from build123d import *

# Parameters (mm, degrees)
SKETCH1_R                                = 4.25
BOSS_EXTRUDE1_DEPTH                      = 10
BOSS_EXTRUDE2_START                      = -5
BOSS_EXTRUDE2_DEPTH                      = 15
SKETCH3_W                                = 342
SKETCH3_H                                = 10
BOSS_EXTRUDE3_DEPTH                      = 304
CUT_EXTRUDE1_REACH                       = 385.234
BOSS_EXTRUDE4_DEPTH                      = 3
MIRROR5_AT_THE_SECOND_PLANE_COPY_1_DEPTH = 3
BOSS_EXTRUDE5_DEPTH                      = 5
BOSS_EXTRUDE5_DEPTH_BACK                 = 5
BOSS_EXTRUDE6_DEPTH                      = 10
SKETCH10_W                               = 19
SKETCH10_H                               = 21.5
SKETCH10_R                               = 4.25
BOSS_EXTRUDE7_DEPTH                      = 10
CUT_EXTRUDE2_REACH                       = 276.29
SKETCH11_W                               = 2.5
SKETCH11_H                               = 70
MIRROR8_COPY_1_DEPTH                     = 10
MIRROR8_COPY_2_DEPTH                     = 10
MIRROR8_COPY_3_SKETCH_W                  = 19
MIRROR8_COPY_3_SKETCH_H                  = 21.5
MIRROR8_COPY_3_SKETCH_R                  = 4.25
MIRROR8_COPY_3_DEPTH                     = 10
CUT_EXTRUDE5_REACH                       = 415.459
SKETCH14_W                               = 574.948758302
SKETCH14_H                               = 178.61459587
CUT_EXTRUDE6_REACH                       = 276.29
SKETCH15_W                               = 297.993149394
SKETCH15_H                               = 172.333387601


with BuildPart() as part:
    # Sketch1 → Boss-Extrude1 (new body)
    with BuildSketch(Plane(origin=(0, 0, 0), x_dir=(1, 0, 0), z_dir=(0, 1, 0))):
        Polygon((-171, 12.5), (171, 12.5), (171, 0), (171, -12.5), (158, -12.5), (158, 0), (-158, 0), (-158, -12.5), (-171, -12.5), align=None)
        with Locations(Location((-145.5, 6.25, 0), (0, 0, 270))):
            Circle(SKETCH1_R, mode=Mode.SUBTRACT)
        with Locations(Location((145.5, 6.25, 0), (0, 0, 90))):
            Circle(SKETCH1_R, mode=Mode.SUBTRACT)
        with Locations(Location((-25.5, 6.25, 0), (0, 0, 270))):
            Circle(SKETCH1_R, mode=Mode.SUBTRACT)
        with Locations(Location((25.5, 6.25, 0), (0, 0, 270))):
            Circle(SKETCH1_R, mode=Mode.SUBTRACT)
    boss_extrude1 = extrude(amount=BOSS_EXTRUDE1_DEPTH)

    # Sketch2 → Boss-Extrude2 (add)
    with BuildSketch(Plane.XY.offset(12.5).offset(BOSS_EXTRUDE2_START)):
        Polygon((-171, 105), (-171, 0), (-158, 0), (-158, 80), (158, 80), (158, 0), (171, 0), (171, 105), align=None)
    boss_extrude2 = extrude(amount=BOSS_EXTRUDE2_DEPTH)

    # Sketch3 → Boss-Extrude3 (add)
    with BuildSketch(Plane.XY.offset(22.5)):
        with Locations((0, 85)):
            Rectangle(SKETCH3_W, SKETCH3_H)
    extrude(amount=BOSS_EXTRUDE3_DEPTH)

    # Sketch4 → Cut-Extrude1 (cut, up to next)
    with BuildSketch(Plane(origin=(0, 105, 0), x_dir=(1, 0, 0), z_dir=(0, 1, 0)), mode=Mode.PRIVATE) as cut_extrude1_sk1:
        Polygon((-163.5, -22.5), (-5, -22.5), (-5, -326.5), (-163.5, -326.5), (-163.5, -39.75), (-163.5, -34.75), align=None)
    cut_extrude1_tool1 = extrude(cut_extrude1_sk1.sketch, amount=-CUT_EXTRUDE1_REACH, mode=Mode.PRIVATE) & part.part
    # Sketch4 → Cut-Extrude1 (cut, up to next)
    with BuildSketch(Plane(origin=(0, 105, 0), x_dir=(1, 0, 0), z_dir=(0, 1, 0)), mode=Mode.PRIVATE) as cut_extrude1_sk2:
        Polygon((163.5, -22.5), (163.5, -51.4723011), (163.5, -326.5), (5, -326.5), (5, -39.75), (5, -22.5), align=None)
    cut_extrude1_tool2 = extrude(cut_extrude1_sk2.sketch, amount=-CUT_EXTRUDE1_REACH, mode=Mode.PRIVATE) & part.part
    add(cut_extrude1_tool1.solids().sort_by_distance((-84.25, 105, 174.5))[0], mode=Mode.SUBTRACT)
    add(cut_extrude1_tool2.solids().sort_by_distance((84.25, 105, 174.5))[0], mode=Mode.SUBTRACT)

    # Mirror3: Boss-Extrude2 across plane
    add(boss_extrude2.mirror(Plane(origin=(0, 0, 174.5), x_dir=(1, 0, 0), z_dir=(0, 0, -1))))

    # Mirror4: Boss-Extrude1 across plane
    add(boss_extrude1.mirror(Plane(origin=(0, 0, 174.5), x_dir=(1, 0, 0), z_dir=(0, 0, -1))))

    # Sketch7 → Boss-Extrude4 (add)
    with BuildSketch(Plane(origin=(0, 80, 0), x_dir=(-1, 0, 0), z_dir=(0, -1, 0))):
        Polygon((-163.5, -22.5), (-148.5, -22.5), (-163.5, -37.5), align=None)
        Polygon((-5, -22.5), (-20, -22.5), (-5, -37.5), align=None)
    boss_extrude4 = extrude(amount=-BOSS_EXTRUDE4_DEPTH)

    # Mirror5: Boss-Extrude4 across plane
    add(boss_extrude4.mirror(Plane(origin=(0, 0, 174.5), x_dir=(1, 0, 0), z_dir=(0, 0, -1))))

    # Mirror5 at the second plane: Boss-Extrude4 across plane
    add(boss_extrude4.mirror(Plane(origin=(0, 0, 0), x_dir=(0, 0, 1), z_dir=(1, 0, 0))))

    # Mirror5 at the second plane copy 1 sketc → Mirror5 at the second plane copy 1 (add)
    with BuildSketch(Plane(origin=(0, 80, 349), x_dir=(1, 0, 0), z_dir=(0, -1, 0))):
        Polygon((-163.5, -22.5), (-148.5, -22.5), (-163.5, -37.5), align=None)
        Polygon((-5, -22.5), (-20, -22.5), (-5, -37.5), align=None)
    extrude(amount=-MIRROR5_AT_THE_SECOND_PLANE_COPY_1_DEPTH)

    # Sketch8 → Boss-Extrude5 (add, two sides: drawn at the far end of the back side and taken through both)
    with BuildSketch(Plane(origin=(0, 0, 0), x_dir=(0, 0, -1), z_dir=(1, 0, 0)).offset(-BOSS_EXTRUDE5_DEPTH_BACK)):
        Polygon((-326.5, 80), (-341.5, 80), (-341.5, 10), (-349, 10), (-349, 0), (-326.5, 0), align=None)
        Polygon((-22.5, 80), (-7.5, 80), (-7.5, 10), (0, 10), (0, 0), (-22.5, 0), align=None)
    extrude(amount=BOSS_EXTRUDE5_DEPTH + BOSS_EXTRUDE5_DEPTH_BACK)

    # Sketch9 → Boss-Extrude6 (add)
    with BuildSketch(Plane(origin=(0, 0, 174.5), x_dir=(-1, 0, 0), z_dir=(0, 0, -1))):
        Polygon((-163.5, 10), (-136, 10), (-136, 0), (-171, 0), (-171, 80), (-163.5, 80), align=None)
    boss_extrude6 = extrude(amount=BOSS_EXTRUDE6_DEPTH)

    # Sketch10 → Boss-Extrude7 (add)
    with BuildSketch(Plane(origin=(0, 10, 0), x_dir=(1, 0, 0), z_dir=(0, 1, 0))):
        with Locations((145.5, -153.75)):
            Rectangle(SKETCH10_W, SKETCH10_H)
        with Locations(Location((145.5, -153.75, 0), (0, 0, 270))):
            Circle(SKETCH10_R, mode=Mode.SUBTRACT)
    boss_extrude7 = extrude(amount=-BOSS_EXTRUDE7_DEPTH)

    # Mirror6: Boss-Extrude6 across plane
    add(boss_extrude6.mirror(Plane(origin=(85.5, 0, 0), x_dir=(0, 0, 1), z_dir=(1, 0, 0))))

    # Mirror7: Boss-Extrude6, Boss-Extrude7 across plane
    add(boss_extrude6.mirror(Plane(origin=(85.5, 0, 0), x_dir=(0, 0, 1), z_dir=(1, 0, 0))))
    add(boss_extrude7.mirror(Plane(origin=(85.5, 0, 0), x_dir=(0, 0, 1), z_dir=(1, 0, 0))))

    # Sketch11 → Cut-Extrude2 (cut, up to next)
    with BuildSketch(Plane.XY.offset(174.5), mode=Mode.PRIVATE) as cut_extrude2_sk1:
        with Locations((6.25, 45)):
            Rectangle(SKETCH11_W, SKETCH11_H)
    cut_extrude2_tool1 = extrude(cut_extrude2_sk1.sketch, amount=-CUT_EXTRUDE2_REACH, mode=Mode.PRIVATE) & part.part
    cut_extrude2 = cut_extrude2_tool1.solids().sort_by_distance((6.25, 45, 174.5))[0]
    add(cut_extrude2, mode=Mode.SUBTRACT)

    # Mirror8: Boss-Extrude6, Boss-Extrude7 across plane
    add(boss_extrude6.mirror(Plane(origin=(0, 0, 174.5), x_dir=(1, 0, 0), z_dir=(0, 0, -1))))
    add(boss_extrude7.mirror(Plane(origin=(0, 0, 174.5), x_dir=(1, 0, 0), z_dir=(0, 0, -1))))

    # Mirror8 copy 1 sketch → Mirror8 copy 1 (add)
    with BuildSketch(Plane(origin=(171, 0, 174.5), x_dir=(1, 0, 0), z_dir=(0, 0, 1))):
        Polygon((-163.5, 10), (-136, 10), (-136, 0), (-171, 0), (-171, 80), (-163.5, 80), align=None)
    extrude(amount=MIRROR8_COPY_1_DEPTH)

    # Mirror8 copy 2 sketch → Mirror8 copy 2 (add)
    with BuildSketch(Plane(origin=(171, 0, 174.5), x_dir=(1, 0, 0), z_dir=(0, 0, 1))):
        Polygon((-163.5, 10), (-136, 10), (-136, 0), (-171, 0), (-171, 80), (-163.5, 80), align=None)
    extrude(amount=MIRROR8_COPY_2_DEPTH)

    # Mirror8 copy 3 sketch → Mirror8 copy 3 (add)
    with BuildSketch(Plane(origin=(171, 10, 349), x_dir=(-1, 0, 0), z_dir=(0, 1, 0))):
        with Locations((145.5, -153.75)):
            Rectangle(MIRROR8_COPY_3_SKETCH_W, MIRROR8_COPY_3_SKETCH_H)
        with Locations(Location((145.5, -153.75, 0), (0, 0, 270))):
            Circle(MIRROR8_COPY_3_SKETCH_R, mode=Mode.SUBTRACT)
    extrude(amount=-MIRROR8_COPY_3_DEPTH)

    # Mirror9: Cut-Extrude2 across plane
    add(cut_extrude2.mirror(Plane(origin=(0, 0, 174.5), x_dir=(1, 0, 0), z_dir=(0, 0, -1))), mode=Mode.SUBTRACT)

    # Sketch14 → Cut-Extrude5 (cut, up to next)
    with BuildSketch(Plane(origin=(0, 0, 0), x_dir=(0, 0, -1), z_dir=(1, 0, 0)), mode=Mode.PRIVATE) as cut_extrude5_sk1:
        with Locations((-145.651613791, 39.902643452)):
            Rectangle(SKETCH14_W, SKETCH14_H)
    cut_extrude5_tool1 = extrude(cut_extrude5_sk1.sketch, amount=-CUT_EXTRUDE5_REACH, mode=Mode.PRIVATE) & part.part
    add(cut_extrude5_tool1.solids().sort_by_distance((0, 39.902643, 145.651614))[0], mode=Mode.SUBTRACT)

    # Sketch15 → Cut-Extrude6 (cut, up to next)
    with BuildSketch(Plane(origin=(0, 0, 174.5), x_dir=(-1, 0, 0), z_dir=(0, 0, -1)), mode=Mode.PRIVATE) as cut_extrude6_sk1:
        with Locations((-69.086440229, 41.027003033)):
            Rectangle(SKETCH15_W, SKETCH15_H)
    cut_extrude6_tool1 = extrude(cut_extrude6_sk1.sketch, amount=-CUT_EXTRUDE6_REACH, mode=Mode.PRIVATE) & part.part
    add(cut_extrude6_tool1.solids().sort_by_distance((69.08644, 41.027003, 174.5))[0], mode=Mode.SUBTRACT)


solid = part.part
The listing builds one solid part. Answer for the finished solid, in the listing's coordinates (mm). A direction names the side the tool comes from. Give positions to 0.01 mm unless a question says otherwise; leave off trailing zeros. Write each loop counter-clockwise with the first axis right and the second up, starting at its lowest first coordinate (ties: lowest second). Pieces come first, ordered by that corner, then holes. Notation, with made-up numbers: (30.25, -19.5) -> (73.25, -19.5) arc R22 ccw to (73.25, 17.5) -> close; hole circle Ø4 at (36, -5). An arc over 180 degrees is marked (long way). Use a Markdown table: item, result.
(1) Flat-ended cylindrical pins translate along their axes: P1, Ø8, axis at y = 4, z = 154.5, coming from the -X side; P2, Ø4, axis at x = 99, y = 83.5, coming from the +Z side; P3, Ø7, axis at x = 25.5, z = 153.75, coming from the +Y side; P4, Ø13, axis at x = 7.5, y = 30.5, coming from the -Z side. Find the tip coordinate at first contact, or state that the pin passes through.
Return value:
| item | result |
|---|---|
| P1 | x = 16 |
| P2 | z = 22.5 |
| P3 | through |
| P4 | z = 7.5 |
(2) Section C-C, the plane z = 153.75 is taken. Determine the outline of the cut face in (x, y).
Return value:
| item | result |
|---|---|
| outline | (0, 80) -> (5, 80) -> (5, 90) -> (0, 90) -> close; (16, 0) -> (21.25, 0) -> (21.25, 10) -> (16, 10) -> close; (29.75, 0) -> (35, 0) -> (35, 10) -> (29.75, 10) -> close; (136, 0) -> (141.25, 0) -> (141.25, 10) -> (136, 10) -> close; (149.75, 0) -> (155, 0) -> (155, 10) -> (149.75, 10) -> close; (163.5, 80) -> (171, 80) -> (171, 90) -> (163.5, 90) -> close |
(3) Section D-D, the plane z = 119.5 is taken. Determine the outline of the cut face in (x, y), then the cut area to 3 significant figures.
Return value:
| item | result |
|---|---|
| outline | (0, 80) -> (5, 80) -> (5, 90) -> (0, 90) -> close; (163.5, 80) -> (171, 80) -> (171, 90) -> (163.5, 90) -> close |
| area | 125 mm2 |
(4) For faces 4 (the flat face through (159, 83, 27)), 5 (the flat face through (164, 41, 22.5)), 6 (the flat face through (26, 5, 143)), determine the directions among +Z, -Z, +X, -X, +Y, -Y from which every point of the face is accessible in a straight line to the end or side of a thin tool.
Return value:
| item | result |
|---|---|
| face 4 | +Z, +Y |
| face 5 | +X, -X, -Y |
| face 6 | +X, -X, +Y, -Y |
(5) Section B-B, the plane y = 65.5 is taken. Determine the outline of the cut face in (x, z), then the cut area to 3 significant figures.
Return value:
| item | result |
|---|---|
| outline | (0, 7.5) -> (5, 7.5) -> (5, 22.5) -> (0, 22.5) -> close; (0, 164.5) -> (5, 164.5) -> (5, 174.5) -> (0, 174.5) -> close; (158, 7.5) -> (171, 7.5) -> (171, 22.5) -> (158, 22.5) -> close; (163.5, 164.5) -> (171, 164.5) -> (171, 174.5) -> (163.5, 174.5) -> close |
| area | 395 mm2 |
(6) Determine the mould class of faces 1 (the flat face through (136, 5, 159)), 2 (the flat face through (145, 5, 143)), 3 (the flat face through (171, 83, 67)) for opening direction X: released by +X, released by -X, zero draft, split by the parting line, or undercut.
Return value:
| item | result |
|---|---|
| face 1 | undercut |
| face 2 | zero draft |
| face 3 | released by +X |
(7) Section A-A, the plane x = 145.5 is taken. Determine the outline of the cut face in (y, z), then the cut area to 3 significant figures.
Return value:
| item | result |
|---|---|
| outline | (0, -12.5) -> (10, -12.5) -> (10, -10.5) -> (0, -10.5) -> close; (0, -2) -> (10, -2) -> (10, 0) -> (0, 0) -> close; (0, 143) -> (10, 143) -> (10, 149.5) -> (0, 149.5) -> close; (0, 158) -> (10, 158) -> (10, 174.5) -> (0, 174.5) -> close; (80, 7.5) -> (105, 7.5) -> (105, 22.5) -> (80, 22.5) -> close |
| area | 645 mm2 |
(8) Find the intervals of material crossed by probe 1 along X at (y, z) = (3, -6); probe 2 along X at (y, z) = (3.5, 153.75); probe 3 along Z at (x, y) = (145, 7), in increasing order. Write a range as from..to.
Return value:
| item | result |
|---|---|
| probe 1 | 0..21.26, 29.74..141.26, 149.74..171 |
| probe 2 | 16..21.25, 29.75..35, 136..141.25, 149.75..155 |
| probe 3 | -12.5..-10.47, -2.03..0, 143..149.53, 157.97..174.5 |
